from build123d import *

# Parameters (mm, degrees)
BOSS_EXTRUDE1_DEPTH = 31.75
FILLET1_R           = 12.7
CUT_EXTRUDE1_DEPTH  = 63.5
SKETCH5_R           = 30.48
BOSS_EXTRUDE2_DEPTH = 34.925
SKETCH6_R           = 9.525
CUT_EXTRUDE2_DEPTH  = 35.925
SKETCH7_R           = 14.2875
CUT_EXTRUDE3_DEPTH  = 6.35
CUT_EXTRUDE4_DEPTH  = 10.525
BOSS_EXTRUDE6_DEPTH = 3.175
BOSS_EXTRUDE7_DEPTH = 6.35
SKETCH11_R          = 6.35
BOSS_EXTRUDE8_DEPTH = 12.7


with BuildPart() as part:
    # Sketch2 → Boss-Extrude1 (new body, symmetric)
    with BuildSketch(Plane.XY):
        Polygon((0, 0), (0, 9.525), (-120.65, 9.525), (-120.65, 0), (-47.625, 0), (-47.625, 5.715), (-34.925, 5.715), (-34.925, 0), align=None)
    extrude(amount=BOSS_EXTRUDE1_DEPTH, both=True)

    # Fillet1
    fillet1_edges = [part.edges().sort_by_distance(p)[0] for p in [
        (-120.65, 4.7625, -31.75),
        (-120.65, 4.7625, 31.75),
    ]]
    fillet(fillet1_edges, radius=FILLET1_R)

    # Sketch3 → Cut-Extrude1 (cut)
    with BuildSketch(Plane(origin=(0, 9.525, 0), x_dir=(1, 0, 0), z_dir=(0, 1, 0))):
        with BuildLine():
            Line((-107.95, 25.4), (-76.2, 25.4))
            ThreePointArc((-76.2, 25.4), (-69.85, 19.05), (-76.2, 12.7))
            Line((-76.2, 12.7), (-107.95, 12.7))
            ThreePointArc((-107.95, 12.7), (-114.3, 19.05), (-107.95, 25.4))
        make_face()
        with BuildLine():
            Line((-107.95, -25.4), (-76.2, -25.4))
            ThreePointArc((-76.2, -25.4), (-69.85, -19.05), (-76.2, -12.7))
            Line((-76.2, -12.7), (-107.95, -12.7))
            ThreePointArc((-107.95, -12.7), (-114.3, -19.05), (-107.95, -25.4))
        make_face()
    extrude(amount=-CUT_EXTRUDE1_DEPTH, mode=Mode.SUBTRACT)

    # Sketch5 → Boss-Extrude2 (add)
    with BuildSketch(Plane(origin=(0, 0, 0), x_dir=(1, 0, 0), z_dir=(0, 1, 0))):
        Circle(SKETCH5_R)
    extrude(amount=BOSS_EXTRUDE2_DEPTH)

    # Sketch6 → Cut-Extrude2 (cut, through all)
    with BuildSketch(Plane(origin=(0, 34.925, 0), x_dir=(1, 0, 0), z_dir=(0, 1, 0))):
        Circle(SKETCH6_R)
    extrude(amount=-CUT_EXTRUDE2_DEPTH, mode=Mode.SUBTRACT)

    # Sketch7 → Cut-Extrude3 (cut)
    with BuildSketch(Plane(origin=(0, 34.925, 0), x_dir=(1, 0, 0), z_dir=(0, 1, 0))):
        Circle(SKETCH7_R)
    extrude(amount=-CUT_EXTRUDE3_DEPTH, mode=Mode.SUBTRACT)

    # Sketch8 → Cut-Extrude4 (cut, through all)
    with BuildSketch(Plane(origin=(0, 9.525, 0), x_dir=(1, 0, 0), z_dir=(0, 1, 0))):
        with BuildLine():
            Line((-60.325, 31.75), (-24.157536171, 18.586119717))
            ThreePointArc((-24.157536171, 18.586119717), (-13.463384994, 27.345340819), (0, 30.48))
            Line((0, 30.48), (0, 31.75))
            Line((0, 31.75), (-60.325, 31.75))
        make_face()
        with BuildLine():
            Line((0, -31.75), (-60.325, -31.75))
            Line((-60.325, -31.75), (-24.157536171, -18.586119717))
            ThreePointArc((-24.157536171, -18.586119717), (-13.463384994, -27.345340819), (0, -30.48))
            Line((0, -30.48), (0, -31.75))
        make_face()
    extrude(amount=-CUT_EXTRUDE4_DEPTH, mode=Mode.SUBTRACT)

    # Sketch9 → Boss-Extrude6 (add, symmetric)
    with BuildSketch(Plane.XY):
        Polygon((-73.025, 9.525), (-33.02, 34.925), (-28.575, 34.925), (-28.575, 9.525), align=None)
    extrude(amount=BOSS_EXTRUDE6_DEPTH, both=True)

    # Sketch10 → Boss-Extrude7 (add)
    with BuildSketch(Plane(origin=(0, 9.525, 0), x_dir=(1, 0, 0), z_dir=(0, 1, 0))):
        Polygon((-81.809712214, 0), (-86.942356107, 8.89), (-97.207643893, 8.89), (-102.340287786, 0), (-97.207643893, -8.89), (-86.942356107, -8.89), align=None)
    extrude(amount=BOSS_EXTRUDE7_DEPTH)

    # Sketch11 → Boss-Extrude8 (add)
    with BuildSketch(Plane(origin=(0, 15.875, 0), x_dir=(1, 0, 0), z_dir=(0, 1, 0))):
        with Locations((-92.075, 0)):
            Circle(SKETCH11_R)
    extrude(amount=BOSS_EXTRUDE8_DEPTH)


solid = part.part
Check sheet for the modelled part. Datum: model origin and axes. Units: mm. A direction names the side the tool comes from. Give positions to 0.01 mm unless a question says otherwise; leave off trailing zeros. Loops run counter-clockwise (first coordinate to the right, second up) from the corner with the lowest first, then second, coordinate; pieces in that order, holes last. Notation, with made-up numbers: M -39.5,-37 L -17.5,-37 A37 ccw -17.5,1 Z; hole C 17,-10 d1. An arc over 180 degrees is marked long. Answer as a JSON object with one key per item and string values. Group by question number.
Q1. Cross-section at C-C on y = 24. Record the cut outline in (x, z) (3 decimals), then the cut area to 3 significant figures.
Q2. Cross-section at D-D on x = -28.5. Record the cut outline in (y, z) (1 decimal), then the cut area to 3 significant figures.
Q3. Go/stop test with flat-tipped pins: P1, Ø6, axis at x = -41, y = 25, coming from the -Z side (3 decimals); P2, Ø1, axis at x = -8.5, y = 21.5, coming from the -Z side; P3, Ø12.5, axis at x = -55, y = 28, coming from the +Z side (3 decimals); P4, Ø1.5, axis at x = -6, z = -19.5, coming from the -Y side. Record where each tip stops, or that it passes through.
Q4. Access from +Z, -Z, +X, -X, +Y, -Y to the whole of each face (thin tool, end or side, straight path). Record for faces 4 (the flat face through (-34.925, 3, 0)), 5 (the cylindrical face through (-98.42, 22.14, -0.28)), 6 (the cylindrical face through (-69.85, 4.83, -19.19)).
Q5. Cross-section at B-B on x = -52.5. Record the cut outline in (y, z) (3 decimals).
Q6. Material ranges on line 1 along Z through (x, y) = (-106, 7); line 2 along Z through (x, y) = (0, 21.5) (3 decimals); line 3 along X through (y, z) = (23.5, -3.5), recorded low to high. Write a range as [from, to].
Q7. Cross-section at A-A on y = 13.5. Record the cut outline in (x, z) (3 decimals).
Q8. Release check for a two-part mould opening along Y. For faces 1 (the cylindrical face through (-14.274, 31.794, -0.628)), 2 (the flat face through (-41, 5.715, 0)), 3 (the flat face through (-85, 15.875, 0)) record: released by +Y, released by -Y, zero draft, split by the parting line, or undercut.
Evaluation:
{
 "1": {"outline": "C -92.075,0 d12.7; M -50.227,-3.175 L -30.314,-3.175 A30.48 ccw long -30.314,3.175 L -50.227,3.175 Z; hole C 0,0 d19.05", "area": "2,890 mm2"},
 "2": {"outline": "M 0,-20.2 L 9.5,-20.2 L 9.5,-10.8 L 34.9,-10.8 L 34.9,10.8 L 9.5,10.8 L 9.5,20.2 L 0,20.2 Z", "area": "933 mm2"},
 "3": {"P1": "stops at z = -3.175", "P2": "stops at z = -29.41", "P3": "stops at z = 3.175", "P4": "stops at y = 0"},
 "4": {"face 4": "+Z, -Z, -Y", "face 5": "+Y", "face 6": "+Y, -Y"},
 "5": {"outline": "M 0,-28.902 L 9.525,-28.902 L 9.525,-3.175 L 22.557,-3.175 L 22.557,3.175 L 9.525,3.175 L 9.525,28.902 L 0,28.902 Z"},
 "6": {"line 1": "z = [-31.75, -25.4], [-12.7, 12.7], [25.4, 31.75]", "line 2": "z = [-30.48, -9.525], [9.525, 30.48]", "line 3": "x = [-97.37, -86.78], [-30.28, -8.86], [8.86, 30.28]"},
 "7": {"outline": "M -102.34,0 L -97.208,-8.89 L -86.942,-8.89 L -81.81,0 L -86.942,8.89 L -97.208,8.89 Z; M -66.764,-3.175 L -30.314,-3.175 A30.48 ccw long -30.314,3.175 L -66.764,3.175 Z; hole C 0,0 d19.05"},
 "8": {"face 1": "zero draft", "face 2": "released by -Y", "face 3": "released by +Y"}
}
